```python
from build123d import *

# Parameters (mm, degrees)
F0_W     = 336.55
F0_H     = 25.4
F1_DEPTH = 25.4
F2_R     = 12.69999
F3_R     = 6.35
F4_DEPTH = 12.7
F5_R     = 6.35
F6_DEPTH = 25.401


# Not quite as in the source:
# - a fillet or chamfer is up to 0.001 mm smaller than in the source, because OpenCascade refuses the exact size


with BuildPart() as f1:
    # F0 (on Front) → F1 (new body)
    with BuildSketch(Plane.XZ):
        with Locations((29.4598335922, -16.8253869212)):
            Rectangle(F0_W, F0_H)
    extrude(amount=F1_DEPTH)

    # F2 (radius 12.7 in the source; OpenCascade refuses exactly that, so slightly less here)
    f2_edges = [f1.edges().sort_by_distance(p)[0] for p in [
        (-138.815166, -12.7, -4.125387),
        (-138.815166, -12.7, -29.525387),
        (197.734834, -12.7, -29.525387),
        (197.734834, -12.7, -4.125387),
    ]]
    fillet(f2_edges, radius=F2_R)

    # F3 (on face) → F4 (join)
    with BuildSketch(Plane(origin=(0, 0, 0), x_dir=(-1, 0, 0), z_dir=(0, 1, 0))):
        with Locations((126.1151664078, -16.8253869212)):
            Circle(F3_R)
    extrude(amount=F4_DEPTH)

    # F5 (on face) → F6 (cut, through all)
    with BuildSketch(Plane(origin=(0, 0, 0), x_dir=(-1, 0, 0), z_dir=(0, 1, 0))):
        with Locations((-185.0348335922, -16.8253869212)):
            Circle(F5_R)
    extrude(amount=-F6_DEPTH, mode=Mode.SUBTRACT)


solid = f1.part
```
The model under review builds one solid part; all positions refer to its coordinate system, in mm. Round coordinates to 2 decimals unless told otherwise and drop trailing zeros. Order: outer loops, then holes, each group sorted by start corner. A loop starts at its lowest first (then second) coordinate and runs counter-clockwise, first axis right, second up.
(1) Take a section at B-B, the plane x = 106. State the section outline as (y, z) points, plus the area to 3 significant figures.
Working result:
outline: (-25.4, -29.53) - (0, -29.53) - (0, -4.13) - (-25.4, -4.13) - close
area: 645 mm2
(2) Take a section at C-C, the plane z = -26. State the section outline as (x, y) points, plus the area to 3 significant figures.
Working result:
outline: (-134.9, -25.4) - (193.82, -25.4) - (193.82, 0) - (-134.9, 0) - close
area: 8,350 mm2
(3) For P1, Ø4, axis at y = -1, z = -20.5, coming from the -X side; P2, Ø7.5, axis at x = -5, z = -13, coming from the +Y side; P3, Ø8, axis at y = -13.5, z = -23, coming from the +X side, all flat-tipped, find the tip position at first contact; note any pin that passes through.
Working result:
P1: stops at x = -138.7
P2: stops at y = 0
P3: stops at x = 197.55
(4) Wall thickness on L1, parallel to X at y = 6, z = -17.5; L2, parallel to Y at x = 60, z = -7.25; L3, parallel to Z at x = 180.5, y = -5: over which ranges is each line inside the solid? List them lowest first.
Working result:
L1: x = -132.43 to -119.8
L2: y = -25.4 to 0
L3: z = -29.53 to -21.27, -12.38 to -4.13
(5) Mouldability with a two-part tool opening along X and no side actions: class faces 1 (the face through (194.11, -12.88, -7.94)), 2 (the face through (-119.77, 6.26, -16.55)), 3 (the face through (191.38, -12.52, -16.55)), 4 (the face through (27, -13, -29.525)) as released by +X, released by -X, zero draft, split by the parting line, or undercut.
Working result:
face 1: released by +X
face 2: split by the parting line
face 3: undercut
face 4: zero draft
